Check sheet for the modelled part. Datum: model origin and axes. Units: mm. Face numbers are marked on the shaded views. A direction names the side the tool comes from. Give positions to 0.01 mm unless a question says otherwise; leave off trailing zeros. Order: outer loops, then holes, each group sorted by start corner. A loop starts at its lowest first (then second) coordinate and runs counter-clockwise, first axis right, second up.
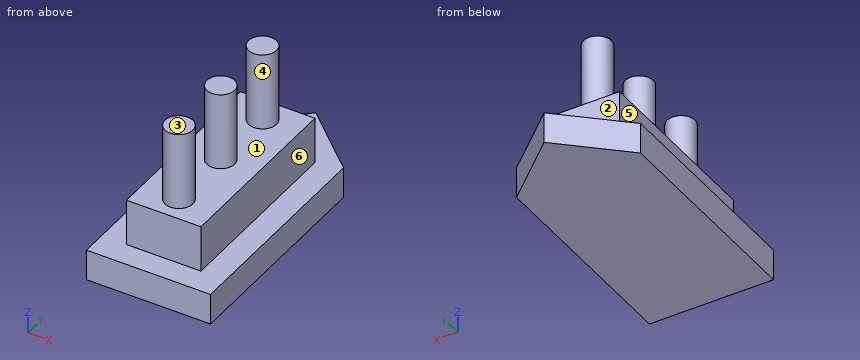
from build123d import *

# Parameters (mm, degrees)
F1_DEPTH = 10
F2_W     = 24
F2_H     = 60
F3_DEPTH = 25
F4_R     = 4.5
F5_DEPTH = 25


with BuildPart() as f1:
    # F0 (on Top) → F1 (new body)
    with BuildSketch(Plane.XY):
        Polygon((0, 53.662619), (-20, 35.524262), (-20, -34.475738), (20, -34.475738), (20, 35.524262), align=None)
    extrude(amount=F1_DEPTH)

    # F2 (on Top) → F3 (join)
    with BuildSketch(Plane.XY):
        with Locations((0, 3.524262)):
            Rectangle(F2_W, F2_H)
    extrude(amount=F3_DEPTH)

    # F4 (on face) → F5 (join)
    with BuildSketch(Plane.XY.offset(25)):
        with Locations((0, 25.524262)):
            Circle(F4_R)
        with Locations((0, 3.524262)):
            Circle(F4_R)
        with Locations((0, -18.475738)):
            Circle(F4_R)
    extrude(amount=F5_DEPTH)


solid = f1.part
1) Section check C-C, the plane z = 8. Record the cut outline in (x, y).
Recorded:
outline: (-20, -34.48) - (20, -34.48) - (20, 35.52) - (0, 53.66) - (-20, 35.52) - close
2) Draft check along Y on the marked faces 1, 2 and 3. Enter one of: +Y half, -Y half, draft (parallel to the pull), parting line (faces both ways), or undercut.
Recorded:
face 1: undercut
face 2: +Y half
face 3: draft
3) Material ranges on L1, parallel to Y at x = -2, z = 47; L2, parallel to Y at x = -1, z = 36; L3, parallel to Z at x = 11, y = 10, recorded low to high.
Recorded:
L1: y = -22.51 to -14.44, -0.51 to 7.56, 21.49 to 29.56
L2: y = -22.86 to -14.09, -0.86 to 7.91, 21.14 to 29.91
L3: z = 0 to 25
4) Depth check by flat-ended pin: pin 1 Ø1 at (x, z) = (3.5, 40) entering from -Y; pin 2 Ø4 at (y, z) = (32.5, 14) entering from +X; pin 3 Ø12 at (x, z) = (4.5, 17.5) entering from -Y. Enter the tip coordinate at first touch or a pass-through.
Recorded:
pin 1: stops at y = -21.83
pin 2: stops at x = 12
pin 3: stops at y = -26.48
5) Section check D-D, the plane z = 26. Record the cut outline in (x, y).
Recorded:
outline: circle Ø9 at (0, -18.48); circle Ø9 at (0, 3.52); circle Ø9 at (0, 25.52)
6) Section check A-A, the plane y = 32. Record the cut outline in (x, z).
Recorded:
outline: (-20, 0) - (20, 0) - (20, 10) - (12, 10) - (12, 25) - (-12, 25) - (-12, 10) - (-20, 10) - close
7) Set-up check for the marked faces 4, 5 and 6: record each of +Z, -Z, +X, -X, +Y, -Y from which the full face is reachable in a straight line by a thin tool's end or side.
Recorded:
face 4: +Z
face 5: +Z, -X, +Y, -Y
face 6: +Z, +X, +Y, -Y
8) Section check B-B, the plane x = -9. Record the cut outline in (y, z).
Recorded:
outline: (-34.48, 0) - (45.5, 0) - (45.5, 10) - (33.52, 10) - (33.52, 25) - (-26.48, 25) - (-26.48, 10) - (-34.48, 10) - close
